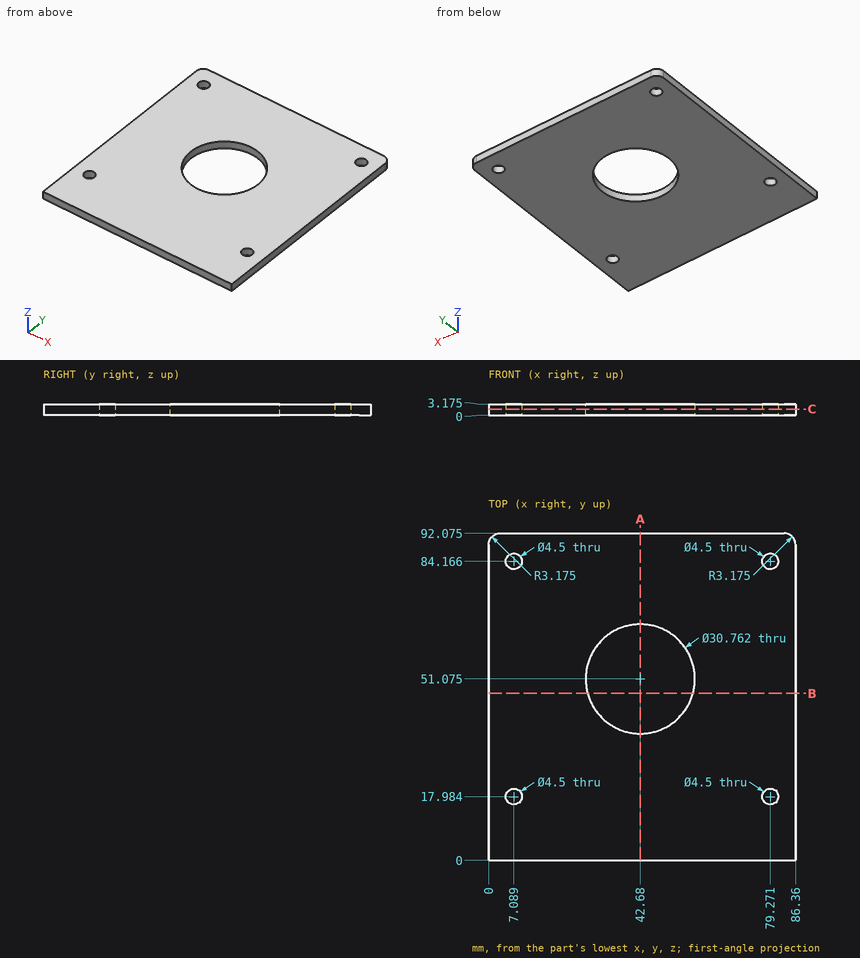
Answer from the drawing. Dimensions are ordinates in mm from the lowest x, y and z of the part. Coordinates: 2 decimals unless noted, no trailing zeros. Write each loop counter-clockwise with the first axis right and the second up, starting at its lowest first coordinate (ties: lowest second). Pieces come first, ordered by that corner, then holes. Notation, with made-up numbers: (48.5, 73) - (104.5, 73) arc R35 ccw to (104.5, 107) - close; hole circle Ø5 at (44, 63). An arc over 180 degrees is marked (long way). Return JSON: item names as keys, results as strings.
1. The part is cut by section B-B on y = 47. Determine the outline of the cut face in (x, z) (1 decimal), then the cut area to 3 significant figures.
Final values:
{"outline": "(0, 0) - (27.8, 0) - (27.8, 3.2) - (0, 3.2) - close; (57.5, 0) - (86.4, 0) - (86.4, 3.2) - (57.5, 3.2) - close", "area": "180 mm^2"}
2. This flat-tipped pin is pushed along its axis until it touches: pin 1 Ø3.5 at (x, y) = (7.09, 17.98) entering from +Z. Where does it stop, or does it pass through?
Final values:
{"pin 1": "through"}
3. Consider line 1 along Y through (x, z) = (42, 0.95) (1 decimal); line 2 along Y through (x, z) = (42.68, 2.3) (1 decimal); line 3 along X through (y, z) = (60.5, 0.3) (1 decimal). Determine where each line is inside the solid, lowest interval first.
Final values:
{"line 1": "0 to 35.7, 66.4 to 92.1", "line 2": "0 to 35.7, 66.5 to 92.1", "line 3": "0 to 30.5, 54.8 to 86.4"}
4. The part is cut by section A-A on x = 42.68. Determine the outline of the cut face in (y, z) (1 decimal), then the cut area to 3 significant figures.
Final values:
{"outline": "(0, 0) - (35.7, 0) - (35.7, 3.2) - (0, 3.2) - close; (66.5, 0) - (92.1, 0) - (92.1, 3.2) - (66.5, 3.2) - close", "area": "195 mm^2"}
5. The part is cut by section C-C on z = 1.7. Count the separate pieces of the cut face and the enclosed holes in it, then the cut area to 3 significant figures.
Final values:
{"separate pieces": "1", "enclosed holes": "5", "area": "7,140 mm^2"}
